The model under review builds one solid part; all positions refer to its coordinate system, in mm. A direction names the side the tool comes from. Round coordinates to 2 decimals unless told otherwise and drop trailing zeros. Loops run counter-clockwise (first coordinate to the right, second up) from the corner with the lowest first, then second, coordinate; pieces in that order, holes last. Notation, with made-up numbers: M -4.75,-9 L 29.25,-9 A30 cw 29.25,17 Z; hole C 52.25,56.25 d10. An arc over 180 degrees is marked long. Use a Markdown table: item, result. Add a question column.
```python
from build123d import *

# Parameters (mm, degrees)
SKETCH1_W           = 59.8
SKETCH1_H           = 37.7
BOSS_EXTRUDE1_DEPTH = 8.9
SKETCH2_W           = 42.2
SKETCH2_H           = 37.7
CUT_EXTRUDE1_DEPTH  = 5.1
SKETCH3_R           = 2.6
CUT_EXTRUDE2_DEPTH  = 49.933730698
SKETCH4_R           = 10
SKETCH4_R_2         = 2.05
CUT_EXTRUDE3_DEPTH  = 36.71193778


with BuildPart() as part:
    # Sketch1 → Boss-Extrude1 (new body)
    with BuildSketch(Plane.XY):
        Rectangle(SKETCH1_W, SKETCH1_H)
    extrude(amount=BOSS_EXTRUDE1_DEPTH)

    # Sketch2 → Cut-Extrude1 (cut)
    with BuildSketch(Plane.XY.offset(8.9)):
        Rectangle(SKETCH2_W, SKETCH2_H)
    extrude(amount=-CUT_EXTRUDE1_DEPTH, mode=Mode.SUBTRACT)

    # Sketch3 → Cut-Extrude2 (cut, through all)
    with BuildSketch(Plane(origin=(0, 18.85, 0), x_dir=(1, 0, 0), z_dir=(0, 1, 0))):
        with Locations(Location((25.5, -4.278740656, 0), (0, 0, 270))):
            Circle(SKETCH3_R)
        with Locations(Location((-25.5, -4.278740656, 0), (0, 0, 90))):
            Circle(SKETCH3_R)
    extrude(amount=-CUT_EXTRUDE2_DEPTH, mode=Mode.SUBTRACT)

    # Sketch4 → Cut-Extrude3 (cut, through all)
    with BuildSketch(Plane.XY.offset(3.8)):
        Circle(SKETCH4_R)
        with Locations((7.957753458, -11.941384338)):
            Circle(SKETCH4_R_2)
        with Locations((-14.320418922, -0.920924483)):
            Circle(SKETCH4_R_2)
        with Locations((6.362665464, 12.862308821)):
            Circle(SKETCH4_R_2)
    extrude(amount=-CUT_EXTRUDE3_DEPTH, mode=Mode.SUBTRACT)


solid = part.part
```
(1) Insertion check: pin 1 Ø3.5 at (x, y) = (6.36, 12.86) entering from +Z; pin 2 Ø6 at (x, y) = (12.5, -8.5) entering from +Z. Each pin has a flat end and moves straight along its axis. Give the tip position at first contact, or say it passes through.
(2) For faces 1 (the face through (29.9, 0, 4)), 2 (the face through (-21.1, 0, 6)), list the 3-axis set-ups (+Z, -Z, +X, -X, +Y, -Y) from which the entire face can be reached by the end or side of a thin tool; tool diameter is ignored.
(3) To check wall thickness, follow probe 1 along X at (y, z) = (-12.5, 4.5); probe 2 along X at (y, z) = (8, 8); probe 3 along Y at (x, z) = (0, 3.05). State the ranges of each line that lie inside material, in increasing order.
(4) Consider section A-A, the plane y = -8. Give the boundary of the cut face in (x, z), then the cut area to 3 significant figures.
(5) Draft analysis for pull direction X (two halves, no side actions). For faces 3 (the face through (-2.17, -9.76, 1.93)), 4 (the face through (-29.9, 0, 4)), 5 (the face through (25, 0, 8.9)), state which applies: released by +X, released by -X, zero draft, split by the parting line, or undercut.
(6) Consider section C-C, the plane z = 8. Give the boundary of the cut face in (x, y).
(7) Consider section B-B, the plane x = -25.5. Give the boundary of the cut face in (y, z).
(8) Consider section D-D, the plane y = 0. Give the boundary of the cut face in (x, z).
Found:
| question | item | result |
|---|---|---|
| 1 | pin 1 | passes through |
| 1 | pin 2 | stops at z = 3.8 |
| 2 | face 1 | +Z, -Z, +X, +Y, -Y |
| 2 | face 2 | +Z, +Y, -Y |
| 3 | probe 1 | x = -29.9 to -28.09, -22.91 to -21.1, 21.1 to 22.91, 28.09 to 29.9 |
| 3 | probe 2 | x = -29.9 to -21.1, 21.1 to 29.9 |
| 3 | probe 3 | y = -18.85 to -10, 10 to 18.85 |
| 4 | outline | M -29.9,0 L -6,0 L -6,3.8 L -21.1,3.8 L -21.1,8.9 L -29.9,8.9 Z; M 6,0 L 29.9,0 L 29.9,8.9 L 21.1,8.9 L 21.1,3.8 L 6,3.8 Z; hole C -25.5,4.28 d5.2; hole C 25.5,4.28 d5.2 |
| 4 | area | 229 mm^2 |
| 5 | face 3 | undercut |
| 5 | face 4 | released by -X |
| 5 | face 5 | zero draft |
| 6 | outline | M -29.9,-18.85 L -21.1,-18.85 L -21.1,18.85 L -29.9,18.85 Z; M 21.1,-18.85 L 29.9,-18.85 L 29.9,18.85 L 21.1,18.85 Z |
| 7 | outline | M -18.85,0 L 18.85,0 L 18.85,1.68 L -18.85,1.68 Z; M -18.85,6.88 L 18.85,6.88 L 18.85,8.9 L -18.85,8.9 Z |
| 8 | outline | M -29.9,0 L -16.15,0 L -16.15,3.8 L -21.1,3.8 L -21.1,8.9 L -29.9,8.9 Z; M -12.49,0 L -10,0 L -10,3.8 L -12.49,3.8 Z; M 10,0 L 29.9,0 L 29.9,8.9 L 21.1,8.9 L 21.1,3.8 L 10,3.8 Z; hole C -25.5,4.28 d5.2; hole C 25.5,4.28 d5.2 |
